Here's how the part is built. I have some questions about the finished solid (model axes, mm). A direction names the side the tool comes from. Coordinates: 2 decimals unless noted, no trailing zeros. Write each loop counter-clockwise with the first axis right and the second up, starting at its lowest first coordinate (ties: lowest second). Pieces come first, ordered by that corner, then holes.
```python
from build123d import *

# Parameters (mm, degrees)
F0_W     = 1.5
F0_H     = 2.806624327
F1_DEPTH = 11.5
F2_DEPTH = 10
F3_DEPTH = 3
F4_DEPTH = 3
F5_DEPTH = 1.5
F6_R     = 4.24999
F7_R     = 2


# Not quite as in the source:
# - a fillet or chamfer is up to 0.001 mm smaller than in the source, because OpenCascade refuses the exact size


with BuildPart() as f1:
    # F0 (on Top) → F1 (new body)
    with BuildSketch(Plane.XY):
        Polygon((-6, 7.25), (-6, 1.443375673), (-6, -1.443375673), (-6, -4.25), (0, -4.25), (0, 7.25), align=None)
        Polygon((-7.5, 4.25), (-7.5, 1.443375673), (-6, 1.443375673), (-6, 7.25), (-7.5, 7.25), align=None)
        Polygon((-7.5, 1.443375673), (-7.5, 1.1999995727), (-7.5, -1.1999995727), (-7.5, -1.443375673), (-6, -1.443375673), (-6, 1.443375673), align=None)
        with Locations((-6.75, -2.8466878365)):
            Rectangle(F0_W, F0_H)
        Polygon((6, 7.25), (0, 7.25), (0, -4.25), (6, -4.25), (6, -1.443375673), (6, 1.443375673), align=None)
        Polygon((7.5, 7.25), (6, 7.25), (6, 1.443375673), (7.5, 1.443375673), (7.5, 4.25), align=None)
        Polygon((7.5, 1.443375673), (6, 1.443375673), (6, -1.443375673), (7.5, -1.443375673), (7.5, -1.1999995727), (7.5, 1.1999995727), align=None)
        with Locations((6.75, -2.8466878365)):
            Rectangle(F0_W, F0_H)
    extrude(amount=F1_DEPTH)

    # F0 (on Top) → F2 (cut)
    with BuildSketch(Plane.XY):
        Polygon((-6, 7.25), (-6, 1.443375673), (-6, -1.443375673), (-6, -4.25), (0, -4.25), (0, 7.25), align=None)
        Polygon((6, 7.25), (0, 7.25), (0, -4.25), (6, -4.25), (6, -1.443375673), (6, 1.443375673), align=None)
    extrude(amount=F2_DEPTH, mode=Mode.SUBTRACT)

    # F0 (on Top) → F3 (cut)
    with BuildSketch(Plane.XY):
        Polygon((-7.5, 1.443375673), (-7.5, 1.1999995727), (-7.5, -1.1999995727), (-7.5, -1.443375673), (-6, -1.443375673), (-6, 1.443375673), align=None)
        Polygon((7.5, 1.443375673), (6, 1.443375673), (6, -1.443375673), (7.5, -1.443375673), (7.5, -1.1999995727), (7.5, 1.1999995727), align=None)
    extrude(amount=F3_DEPTH, mode=Mode.SUBTRACT)

    # F0 (on Top) → F4 (join)
    with BuildSketch(Plane.XY):
        Polygon((-9, 2.3094010768), (-7.5, 1.443375673), (-7.5, 4.25), (-13.3, 4.25), (-13.3, -4.25), (-7.5, -4.25), (-7.5, -1.443375673), (-9, -2.3094010768), (-11, -1.1547005384), (-11, 1.1547005384), align=None)
        Polygon((7.5, -1.443375673), (7.5, -4.25), (13.3, -4.25), (13.3, 4.25), (7.5, 4.25), (7.5, 1.443375673), (9, 2.3094010768), (11, 1.1547005384), (11, -1.1547005384), (9, -2.3094010768), align=None)
    extrude(amount=F4_DEPTH)

    # F0 (on Top) → F5 (join)
    with BuildSketch(Plane.XY):
        with BuildLine():
            ThreePointArc((-9, -1.1999995727), (-10.1999995727, 0), (-9, 1.1999995727))
            Line((-9, 1.1999995727), (-7.5, 1.1999995727))
            Line((-7.5, 1.1999995727), (-7.5, 1.443375673))
            Line((-7.5, 1.443375673), (-9, 2.3094010768))
            Line((-9, 2.3094010768), (-11, 1.1547005384))
            Line((-11, 1.1547005384), (-11, -1.1547005384))
            Line((-11, -1.1547005384), (-9, -2.3094010768))
            Line((-9, -2.3094010768), (-7.5, -1.443375673))
            Line((-7.5, -1.443375673), (-7.5, -1.1999995727))
            Line((-7.5, -1.1999995727), (-9, -1.1999995727))
        make_face()
        with BuildLine():
            Line((9, 2.3094010768), (7.5, 1.443375673))
            Line((7.5, 1.443375673), (7.5, 1.1999995727))
            Line((7.5, 1.1999995727), (9, 1.1999995727))
            ThreePointArc((9, 1.1999995727), (10.1999995727, 0), (9, -1.1999995727))
            Line((9, -1.1999995727), (7.5, -1.1999995727))
            Line((7.5, -1.1999995727), (7.5, -1.443375673))
            Line((7.5, -1.443375673), (9, -2.3094010768))
            Line((9, -2.3094010768), (11, -1.1547005384))
            Line((11, -1.1547005384), (11, 1.1547005384))
            Line((11, 1.1547005384), (9, 2.3094010768))
        make_face()
    extrude(amount=F5_DEPTH)

    # F6 (radius 4.25 in the source; OpenCascade refuses exactly that, so slightly less here)
    f6_edges = [f1.edges().sort_by_distance(p)[0] for p in [
        (-13.3, -4.25, 1.5),
        (-13.3, 4.25, 1.5),
        (13.3, 4.25, 1.5),
        (13.3, -4.25, 1.5),
    ]]
    fillet(f6_edges, radius=F6_R)

    # F7
    f7_edges = [f1.edges().sort_by_distance(p)[0] for p in [
        (6, 1.5, 10),
        (7.5, 1.5, 11.5),
        (-7.5, 1.5, 11.5),
        (-6, 1.5, 10),
    ]]
    fillet(f7_edges, radius=F7_R)


solid = f1.part
```
1) Will these pins go through, and if not, where does the flat tip stop? pin 1 (1 mm diameter, centred on y = 4, z = 6.5, fed in from -X); pin 2 (6 mm diameter, centred on y = 5, z = 3, fed in from -X); pin 3 (1.7 mm diameter, centred on x = 12, y = -2, fed in from +Z).
Values follow:
pin 1: stops at x = -7.5
pin 2: stops at x = -12.8
pin 3: stops at z = 3
2) Imagine slicing it at C-C on x = -1.25. Please give me the cut outline in (y, z), then the cut area to 4 significant figures.
Values follow:
outline: (-4.25, 10) - (7.25, 10) - (7.25, 11.5) - (-4.25, 11.5) - close
area: 17.25 mm2
3) Imagine slicing it at B-B on y = 0.25. Please give me the cut outline in (x, z), then the cut area to 3 significant figures.
Values follow:
outline: (-13.29, 0) - (-10.17, 0) - (-10.17, 1.5) - (-11, 1.5) - (-11, 3) - (-13.29, 3) - close; (-7.5, 3) - (-6, 3) - (-6, 8) arc R2 cw to (-4, 10) - (4, 10) arc R2 cw to (6, 8) - (6, 3) - (7.5, 3) - (7.5, 9.5) arc R2 ccw to (5.5, 11.5) - (-5.5, 11.5) arc R2 ccw to (-7.5, 9.5) - close; (10.17, 0) - (13.29, 0) - (13.29, 3) - (11, 3) - (11, 1.5) - (10.17, 1.5) - close
area: 59.7 mm2
4) Imagine slicing it at D-D on z = 9. Please give me the cut outline in (x, y).
Values follow:
outline: (-7.5, -4.25) - (-5.73, -4.25) - (-5.73, 7.25) - (-7.5, 7.25) - close; (5.73, -4.25) - (7.5, -4.25) - (7.5, 7.25) - (5.73, 7.25) - close
5) I need wall thicknesses on probe 1 along X at (y, z) = (-0.5, 6.5); probe 2 along Z at (x, y) = (-0.25, 1); probe 3 along Z at (x, y) = (-8.25, -3.25). Which ranges of each line are inside material? Lowest first, please.
Values follow:
probe 1: x = -7.5 to -6, 6 to 7.5
probe 2: z = 10 to 11.5
probe 3: z = 0 to 3
6) Imagine slicing it at A-A on z = 4.5. Please give me the cut outline in (x, y).
Values follow:
outline: (-7.5, -4.25) - (-6, -4.25) - (-6, 7.25) - (-7.5, 7.25) - close; (6, -4.25) - (7.5, -4.25) - (7.5, 7.25) - (6, 7.25) - close
7) We'd pull the mould along Y, two halves only. Please class faces 1 (the face through (-8.26, 1.88, 2.24)), 2 (the face through (0, -4.25, 10.4)), 3 (the face through (7.5, 1, 6)): pulls with the +Y half, pulls with the -Y half, needs draft (parallel to the pull), parting line crosses it, or undercut.
Values follow:
face 1: undercut
face 2: pulls with the -Y half
face 3: needs draft
8) On a 3-axis mill with a long thin cutter (end or side, diameter ignored), from which of +Z, -Z, +X, -X, +Y, -Y can I reach the whole of each face in a straight line? I mean faces 4 (the face through (-12, 0, 3)), 5 (the face through (-7, 0, 3)), 6 (the face through (8, -1.2, 1)), 7 (the face through (8, 4.25, 1)). Say none if no direction works.
Values follow:
face 4: +Z, -X, +Y, -Y
face 5: -Z
face 6: +Z, -Z
face 7: +Z, -Z, +X, +Y
